Verification items for the finished model (mm, model axes). A direction names the side the tool comes from. Round coordinates to 2 decimals unless told otherwise and drop trailing zeros. Write each loop counter-clockwise with the first axis right and the second up, starting at its lowest first coordinate (ties: lowest second). Pieces come first, ordered by that corner, then holes. Notation, with made-up numbers: (2.5, -11.5) - (14.5, -11.5) arc R12 cw to (14.5, 11.5) - close; hole circle Ø4 at (74.5, 25). An arc over 180 degrees is marked (long way). Answer as a JSON object with one key per item and string values.
```python
from build123d import *

# Parameters (mm, degrees)
F1_ANGLE_BACK  = 30
F1_ANGLE       = 60
F3_D           = 4.5
F3_CBORE_D     = 8
F3_CBORE_DEPTH = 4.5
F4_COUNT       = 6
F8_R           = 3
F9_DEPTH       = 25


with BuildPart() as f1:
    # F0 (on Front) → F1 (revolve)
    with BuildSketch(Plane.XZ, mode=Mode.PRIVATE) as f1_sk:
        Polygon((8, 50), (8, 0), (24.5, 0), (24.5, 10), (15, 10), (15, 50), align=None)
    revolve(f1_sk.sketch.rotate(Axis((0, 0, 41.6573854163), (0, 0, 1)), -F1_ANGLE_BACK), axis=Axis((0, 0, 41.6573854163), (0, 0, 1)), revolution_arc=F1_ANGLE)

    # F3 (through all)
    with Locations(Plane(origin=(0, 0, 0), x_dir=(1, 0, 0), z_dir=(0, 0, -1))):
        with Locations((19.5, 0)):
            CounterBoreHole(F3_D / 2, F3_CBORE_D / 2, F3_CBORE_DEPTH)


with BuildPart() as f4_1:
    # F4: instance of F1
    add(f1.part.rotate(Axis((0, 0, 41.6573854163), (0, 0, -1)), 1 * 360 / F4_COUNT))


with BuildPart() as f4_2:
    # F4: instance of F1
    add(f1.part.rotate(Axis((0, 0, 41.6573854163), (0, 0, -1)), 2 * 360 / F4_COUNT))


with BuildPart() as f4_3:
    # F4: instance of F1
    add(f1.part.rotate(Axis((0, 0, 41.6573854163), (0, 0, -1)), 3 * 360 / F4_COUNT))


with BuildPart() as f4_4:
    # F4: instance of F1
    add(f1.part.rotate(Axis((0, 0, 41.6573854163), (0, 0, -1)), 4 * 360 / F4_COUNT))


with BuildPart() as f4_5:
    # F4: instance of F1
    add(f1.part.rotate(Axis((0, 0, 41.6573854163), (0, 0, -1)), 5 * 360 / F4_COUNT))


with BuildPart() as f4_1_1:
    add(f4_1.part)

    # F5: union F1, F4_5, F4_4, F4_3, F4_2
    add(f1.part)
    add(f4_5.part)
    add(f4_4.part)
    add(f4_3.part)
    add(f4_2.part)

    # F8 (on plane+point) → F9 (cut)
    with BuildSketch(Plane.XZ.offset(-24.5)):
        with Locations((0, 5)):
            Circle(F8_R)
    extrude(amount=F9_DEPTH, mode=Mode.SUBTRACT)


solid = f4_1_1.part
```
Q1. Material ranges on line 1 along X through (y, z) = (18, 7); line 2 along Y through (x, z) = (9.75, 2.7); line 3 along Y through (x, z) = (9, 8), recorded low to high. Write a range as [from, to].
Geometry check:
{"line 1": "x = [-16.62, -11.71], [-7.79, -2.24], [2.24, 7.79], [11.71, 16.62]", "line 2": "y = [-22.48, -20.89], [-12.89, 12.89], [20.89, 22.48]", "line 3": "y = [-22.79, -19.01], [-14.77, 14.77], [19.01, 22.79]"}
Q2. Release check for a two-part mould opening along X. For faces 1 (the cylindrical face through (-4.506, 14.307, 30.28)), 2 (the flat face through (-4, -15, 10)), 3 (the cylindrical face through (16.3, 2.4, 2.2)) record: released by +X, released by -X, zero draft, split by the parting line, or undercut.
Geometry check:
{"face 1": "split by the parting line", "face 2": "zero draft", "face 3": "undercut"}
Q3. Section check A-A, the plane x = 0. Record the cut outline in (y, z), then the cut area to 3 significant figures.
Geometry check:
{"outline": "(-24.5, 0) - (-8, 0) - (-8, 50) - (-15, 50) - (-15, 10) - (-24.5, 10) - close; (8, 0) - (24.5, 0) - (24.5, 2) - (8, 2) - close; (8, 8) - (24.5, 8) - (24.5, 10) - (15, 10) - (15, 50) - (8, 50) - close", "area": "791 mm2"}
Q4. Section check C-C, the plane z = 6. State how many separate pieces and enclosed holes the cut face has, then the cut area to 3 significant figures.
Geometry check:
{"separate pieces": "1", "enclosed holes": "6", "area": "1,500 mm2"}
Q5. Section check B-B, the plane y = 0. Record the cut outline in (x, z).
Geometry check:
{"outline": "(-24.5, 0) - (-23.5, 0) - (-23.5, 4.5) - (-21.75, 4.5) - (-21.75, 10) - (-24.5, 10) - close; (-17.25, 4.5) - (-15.5, 4.5) - (-15.5, 0) - (-8, 0) - (-8, 50) - (-15, 50) - (-15, 10) - (-17.25, 10) - close; (8, 0) - (15.5, 0) - (15.5, 4.5) - (17.25, 4.5) - (17.25, 10) - (15, 10) - (15, 50) - (8, 50) - close; (21.75, 4.5) - (23.5, 4.5) - (23.5, 0) - (24.5, 0) - (24.5, 10) - (21.75, 10) - close"}
Q6. Gauge pin test, flat ends, axial feed: P1, Ø5, axis at x = -19.5, y = 0, coming from the +Z side; P2, Ø12, axis at x = 11, y = 7, coming from the -Z side; P3, Ø1.5, axis at x = 7, z = 34, coming from the +Y side; P4, Ø3.5, axis at x = -9.75, y = -16.89, coming from the +Z side (3 decimals). Record the tip position at first contact, or that the pin passes through.
Geometry check:
{"P1": "stops at z = 10", "P2": "stops at z = 0", "P3": "stops at y = 13.64", "P4": "passes through"}
Q7. Section check D-D, the plane x = 18. Record the cut outline in (y, z).
Geometry check:
{"outline": "(-16.62, 0) - (-3.71, 0) - (-3.71, 4.5) - (-1.68, 4.5) - (-1.68, 10) - (-16.62, 10) - close; (1.68, 4.5) - (3.71, 4.5) - (3.71, 0) - (16.62, 0) - (16.62, 10) - (1.68, 10) - close"}
Q8. Set-up check for faces 4 (the cylindrical face through (12.92, 14.45, 2.22)), 5 (the cylindrical face through (-10.788, -14.891, 7.288)): record each of +Z, -Z, +X, -X, +Y, -Y from which the full face is reachable in a straight line by a thin tool's end or side.
Geometry check:
{"face 4": "-Z", "face 5": "+Z, -Z"}
